from build123d import *

# Parameters (mm, degrees)
F0_W     = 88.9
F0_H     = 139.7
F1_DEPTH = 787.4
F3_DEPTH = 88.9
F4_W     = 50.8
F4_H     = 88.9
F5_DEPTH = 88.9


with BuildPart() as f1:
    # F0 (on Top) → F1 (new body)
    with BuildSketch(Plane.XY):
        with Locations((44.45, 69.85)):
            Rectangle(F0_W, F0_H)
    extrude(amount=F1_DEPTH)

    # F2 (on face) → F3 (cut)
    with BuildSketch(Plane.XY.offset(787.4)):
        Polygon((0, 88.9), (0, 0), (13.611819, 50.8), (75.288181, 50.8), (88.9, 0), (88.9, 88.9), align=None)
    extrude(amount=-F3_DEPTH, mode=Mode.SUBTRACT)

    # F4 (on face) → F5 (cut, through all)
    with BuildSketch(Plane(origin=(0, 0, 0), x_dir=(0, -1, 0), z_dir=(-1, 0, 0))):
        with Locations((-69.85, 273.05)):
            Rectangle(F4_W, F4_H)
    extrude(amount=-F5_DEPTH, mode=Mode.SUBTRACT)


solid = f1.part
Build history of the part. All positions in model axes, mm. A direction names the side the tool comes from. Round coordinates to 2 decimals unless told otherwise and drop trailing zeros. Write each loop counter-clockwise with the first axis right and the second up, starting at its lowest first coordinate (ties: lowest second). Pieces come first, ordered by that corner, then holes. Notation, with made-up numbers: (-24.75, 15) -> (20.25, 15) arc R20 cw to (20.25, 34) -> close; hole circle Ø4 at (35, 26). An arc over 180 degrees is marked (long way). Use one line per item in the form item = value.
Q1. Two-plate mould, pull along Y, no slides. Class faces 1 (the flat face through (44, 139.7, 388)), 2 (the flat face through (0, 69, 388)), 3 (the flat face through (44, 0, 388)), 4 (the flat face through (44, 70, 317.5)): released by +Y, released by -Y, zero draft, split by the parting line, or undercut.
Conclusion:
face_1 = released by +Y
face_2 = zero draft
face_3 = released by -Y
face_4 = undercut
Q2. Band-saw the part on A-A, the plane z = 252. Write the cut outline in (x, y).
Conclusion:
outline = (0, 0) -> (88.9, 0) -> (88.9, 44.45) -> (0, 44.45) -> close; (0, 95.25) -> (88.9, 95.25) -> (88.9, 139.7) -> (0, 139.7) -> close
Q3. Band-saw the part on C-C, the plane x = 52.5. Write the cut outline in (y, z), then the cut area to 3 significant figures.
Conclusion:
outline = (0, 0) -> (139.7, 0) -> (139.7, 787.4) -> (88.9, 787.4) -> (88.9, 698.5) -> (50.8, 698.5) -> (50.8, 787.4) -> (0, 787.4) -> close; hole (44.45, 228.6) -> (95.25, 228.6) -> (95.25, 317.5) -> (44.45, 317.5) -> close
area = 102,000 mm²
Q4. Tool access for faces 5 (the flat face through (44, 44.45, 272)), 6 (the flat face through (81.999, 25.756, 743.572)), 7 (the flat face through (88.9, 69, 388)), 8 (the flat face through (45, 88.9, 744)), 9 (the flat face through (6.7, 25, 743.6)): list every direction of +Z, -Z, +X, -X, +Y, -Y with a clear straight run to the whole face (end or side of a thin tool).
Conclusion:
face_5 = +X, -X
face_6 = +Z, +X
face_7 = +Z, -Z, +X, +Y, -Y
face_8 = +Z, +X, -X
face_9 = +Z, -X
Q5. Band-saw the part on B-B, the plane y = 76. Write the cut outline in (x, z), then the cut area to 3 significant figures.
Conclusion:
outline = (0, 0) -> (88.9, 0) -> (88.9, 228.6) -> (0, 228.6) -> close; (0, 317.5) -> (88.9, 317.5) -> (88.9, 698.5) -> (0, 698.5) -> close
area = 54,200 mm²
Q6. Drill centre lines: L1, parallel to Z at x = 12.5, y = 52.5; L2, parallel to Y at x = 51.5, z = 280.5. Where is each one in solid material? Low to high.
Conclusion:
L1 = 0 to 228.6, 317.5 to 698.5
L2 = 0 to 44.45, 95.25 to 139.7
Q7. Drop flat-ended pins along their axis: P1, Ø6, axis at y = 58, z = 532, coming from the -X side; P2, Ø1.5, axis at x = 22.5, y = 82, coming from the +Z side. Give the stop position or say it passes through.
Conclusion:
P1 = 0
P2 = 698.5
